```python
from build123d import *

# Parameters (mm, degrees)
SKETCH3_R           = 2.5
BOSS_EXTRUDE1_DEPTH = 10
CUT_EXTRUDE2_DEPTH  = 3


with BuildPart() as part:
    # Sketch1 → Revolve1 (revolve)
    with BuildSketch(Plane.XY, mode=Mode.PRIVATE) as revolve1_sk:
        Polygon((-2.5, 0), (0, 0), (0, 1.5), (-3.75, 1.5), (-4.5, 1.2), (-4.5, 0), align=None)
    revolve(revolve1_sk.sketch.rotate(Axis((0, 0, 0), (0, 1, 0)), 270), axis=Axis((0, 0, 0), (0, 1, 0)))

    # Sketch3 → Boss-Extrude1 (add)
    with BuildSketch(Plane.XZ):
        with Locations(Location((0, 0, 0), (0, 0, 90))):
            Circle(SKETCH3_R)
    extrude(amount=BOSS_EXTRUDE1_DEPTH)

    # Sketch2 → Cut-Extrude2 (cut)
    with BuildSketch(Plane(origin=(0, 1.5, 0), x_dir=(1, 0, 0), z_dir=(0, 1, 0))):
        Polygon((1.732050808, 0), (0.866025404, 1.5), (-0.866025404, 1.5), (-1.732050808, 0), (-0.866025404, -1.5), (0.866025404, -1.5), align=None)
    extrude(amount=-CUT_EXTRUDE2_DEPTH, mode=Mode.SUBTRACT)


solid = part.part
```
Here's how the part is built. I have some questions about the finished solid (model axes, mm). A direction names the side the tool comes from. Coordinates: 2 decimals unless noted, no trailing zeros. Order: outer loops, then holes, each group sorted by start corner. A loop starts at its lowest first (then second) coordinate and runs counter-clockwise, first axis right, second up. Notation, with made-up numbers: (80, 35.25) - (133, 35.25) arc R15 cw to (133, 48.25) - close; hole circle Ø11 at (72, 19.25). An arc over 180 degrees is marked (long way). One line per question, with ' | ' between items. Start each with the question number.
1. I'm going to push flat-ended pins straight in: pin 1 Ø0.5 at (x, y) = (-0.5, -0.5) entering from -Z; pin 2 Ø4 at (y, z) = (-7.5, 0.5) entering from +X; pin 3 Ø1 at (x, y) = (-2, -4) entering from +Z. Where does each tip first touch, or does it pass through?
2. If we section it at A-A (x = 0): Write out the boundary of the cut face in (y, z).
3. If we section it at B-B (y = -2.75): Write out the boundary of the cut face in (x, z).
4. If we mould it in two halves opening along Z, with no side actions, what happens to faces 1 (the flat face through (-1.305, 0.021, 0.74)), 2 (the cylindrical face through (-1.352, 0.592, -4.292)), 3 (the flat face through (2, 0, -2))? For each: released by +Z, released by -Z, zero draft, split by the parting line, or undercut.
5. Please list where these lines run through material, in increasing order: line 1 along Y through (x, z) = (-2.5, -1.5); line 2 along Y through (x, z) = (0.75, 0); line 3 along X through (y, z) = (0.25, 0.75). Write a range as [from, to].
6. Which directions (+Z, -Z, +X, -X, +Y, -Y) give clear straight access to the entire face, cutting with the end or side of a thin tool? Please do faces 4 (the cylindrical face through (2.44, -4.93, -0.54)), 5 (the flat face through (0, 1.5, 2)), 6 (the flat face through (0, 0, -1.5)).
Model answer:
1) pin 1: stops at z = -2.49 | pin 2: stops at x = 2.5 | pin 3: stops at z = 2
2) outline: (-10, -2.5) - (0, -2.5) - (0, -4.5) - (1.2, -4.5) - (1.5, -3.75) - (1.5, -1.5) - (-1.5, -1.5) - (-1.5, 1.5) - (1.5, 1.5) - (1.5, 3.75) - (1.2, 4.5) - (0, 4.5) - (0, 2.5) - (-10, 2.5) - close
3) outline: circle Ø5 at (0, 0)
4) face 1: undercut | face 2: split by the parting line | face 3: zero draft
5) line 1: y = [0, 1.5] | line 2: y = [-10, -1.5] | line 3: x = [-4.44, -1.3], [1.3, 4.44]
6) face 4: -Y | face 5: +Z, -Z, +X, -X, +Y | face 6: +Y
